CAD build for the part. Positions are in the model's coordinates, mm. Face numbers are marked on the shaded views. Give positions to 0.01 mm unless a question says otherwise; leave off trailing zeros. Loops run counter-clockwise (first coordinate to the right, second up) from the corner with the lowest first, then second, coordinate; pieces in that order, holes last. Notation, with made-up numbers: (55.25, 76.5) - (92.25, 76.5) arc R9 cw to (92.25, 85.5) - close; hole circle Ø3 at (89, 54). An arc over 180 degrees is marked (long way). Return JSON: item names as keys, results as strings.
from build123d import *

# Parameters (mm, degrees)
BOX072_W     = 20
BOX072_H     = 10
BOX072_DEPTH = 10
BOX071_W     = 50
BOX071_H     = 50
BOX071_DEPTH = 50


with BuildPart() as cubo001:
    # Box072 → Box072 (new body)
    with BuildSketch(Plane(origin=(15, -5, 9), x_dir=(1, 0, 0), z_dir=(0, 0, 1))):
        with Locations((10, 5)):
            Rectangle(BOX072_W, BOX072_H)
    extrude(amount=BOX072_DEPTH)


with BuildPart() as esfera001:
    # Sphere001 → Sphere001 (revolve)
    with BuildSketch(Plane(origin=(37, 2, 35), x_dir=(1, 0, 0), z_dir=(0, -1, 0))):
        with BuildLine():
            ThreePointArc((0, -5), (5, 0), (0, 5))
            Line((0, 5), (0, -5))
        make_face()
    revolve(axis=Axis((37, 2, 35), (0, 0, 1)))


with BuildPart() as esfera:
    # Sphere → Sphere (revolve)
    with BuildSketch(Plane(origin=(13, 2, 35), x_dir=(1, 0, 0), z_dir=(0, -1, 0))):
        with BuildLine():
            ThreePointArc((0, -5), (5, 0), (0, 5))
            Line((0, 5), (0, -5))
        make_face()
    revolve(axis=Axis((13, 2, 35), (0, 0, 1)))


with BuildPart() as cut117:
    # Box071 → Box071 (new body)
    with BuildSketch(Plane.XY):
        with Locations((25, 25)):
            Rectangle(BOX071_W, BOX071_H)
    extrude(amount=BOX071_DEPTH)

    # Cut115: cut Esfera
    add(esfera.part, mode=Mode.SUBTRACT)

    # Cut116: cut Esfera001
    add(esfera001.part, mode=Mode.SUBTRACT)

    # Cut117: cut Cubo001
    add(cubo001.part, mode=Mode.SUBTRACT)


with BuildPart() as cut117_1:
    # Cut117 placement: moved
    add(cut117.part.moved(Location((0, -9, 1))))


solid = cut117_1.part
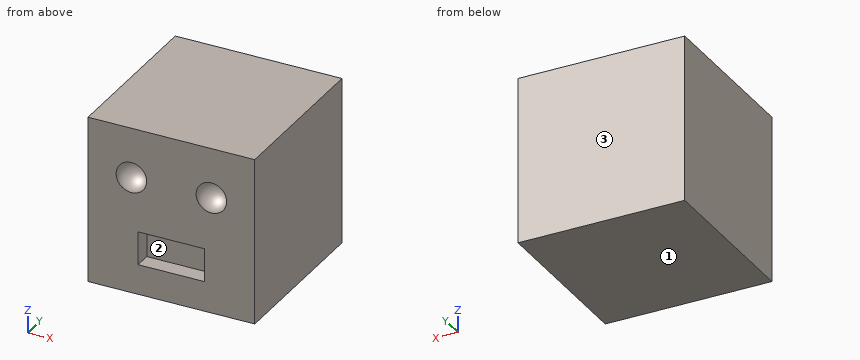
1. Cut at B-B, the plane z = 18. Write the cut outline in (x, y), plus the area to 3 significant figures.
Values follow:
{"outline": "(0, -9) - (15, -9) - (15, -4) - (35, -4) - (35, -9) - (50, -9) - (50, 41) - (0, 41) - close", "area": "2,400 mm²"}
2. Cut at C-C, the plane x = 44.5. Write the cut outline in (y, z).
Values follow:
{"outline": "(-9, 1) - (41, 1) - (41, 51) - (-9, 51) - close"}
3. Drill centre lines: probe 1 along Y at (x, z) = (4, 5.5); probe 2 along Y at (x, z) = (16.5, 17). Where is each one in solid material? Low to high.
Values follow:
{"probe 1": "y = -9 to 41", "probe 2": "y = -4 to 41"}
4. Pull direction Z, two halves, no side cores. Call the marked faces 1, 2 and 3: +Z half, -Z half, draft (parallel to the pull), parting line (faces both ways), or undercut.
Values follow:
{"face 1": "-Z half", "face 2": "undercut", "face 3": "draft"}
5. Cut at A-A, the plane x = 19.5. Write the cut outline in (y, z).
Values follow:
{"outline": "(-9, 1) - (41, 1) - (41, 51) - (-9, 51) - (-9, 20) - (-4, 20) - (-4, 10) - (-9, 10) - close"}
6. Cut at D-D, the plane z = 29. Write the cut outline in (x, y), plus the area to 3 significant figures.
Values follow:
{"outline": "(0, -9) - (50, -9) - (50, 41) - (0, 41) - close", "area": "2,500 mm²"}
7. Drop flat-ended pins along their axis: P1, Ø1, axis at x = 43.5, z = 14, coming from the -Y side; P2, Ø3, axis at x = 29, z = 13.5, coming from the -Y side. Give the stop position or say it passes through.
Values follow:
{"P1": "stops at y = -9", "P2": "stops at y = -4"}
